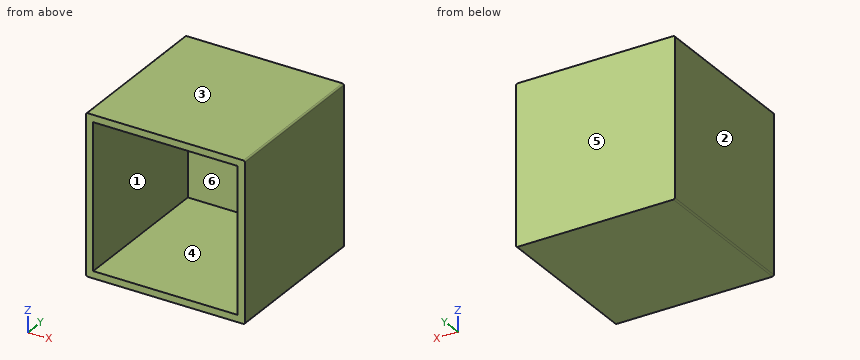
from build123d import *

# Parameters (mm, degrees)
F0_W     = 61.1250735819
F0_H     = 72.7862343192
F1_DEPTH = 28.448
F2_DEPTH = 32.6771
F3_DEPTH = 41.03624
F4_R     = 0.254
F5_T     = -1.27
F6_DEPTH = 3.302


with BuildPart() as f1:
    # F0 (on Top) → F1 (new body)
    with BuildSketch(Plane.XY):
        Rectangle(F0_W, F0_H)
    extrude(amount=F1_DEPTH)

    # F2 (cut): a face of the model
    f2_faces = [f1.faces().sort_by_distance(p)[0] for p in [
        (30.562536791, 0, 14.224),
    ]]
    extrude(f2_faces, amount=-F2_DEPTH, mode=Mode.SUBTRACT)

    # F3 (cut): a face of the model
    f3_faces = [f1.faces().sort_by_distance(p)[0] for p in [
        (-16.33855, -36.3931171596, 14.224),
    ]]
    extrude(f3_faces, amount=-F3_DEPTH, mode=Mode.SUBTRACT)

    # F4
    f4_edges = [f1.edges().sort_by_distance(p)[0] for p in [
        (-2.114563, 20.51812, 28.448),
        (-30.562537, 20.51812, 28.448),
        (-2.114563, 20.51812, 0),
        (-30.562537, 20.51812, 0),
    ]]
    fillet(f4_edges, radius=F4_R)

    # F5
    f5_openings = [f1.faces().sort_by_distance(p)[0] for p in [
        (-16.33855, 4.643123, 14.224),
    ]]
    offset(amount=F5_T, openings=f5_openings)

    # F6 (cut): a face of the model
    f6_faces = [f1.faces().sort_by_distance(p)[0] for p in [
        (-16.33855, 4.6431228404, 0.4023152874),
    ]]
    extrude(f6_faces, amount=-F6_DEPTH, mode=Mode.SUBTRACT)


solid = f1.part
Design review of the part built by this model. Coordinates are the model's own, in mm. Face numbers are marked on the shaded views. A direction names the side the tool comes from. Coordinates: 2 decimals unless noted, no trailing zeros. Order: outer loops, then holes, each group sorted by start corner. A loop starts at its lowest first (then second) coordinate and runs counter-clockwise, first axis right, second up. Notation, with made-up numbers: (3, 2) -> (19, 2) arc R19 ccw to (19, 23) -> close; hole circle Ø5 at (10, 2). An arc over 180 degrees is marked (long way). One line per item, written item: value.
1) We need section B-B, the plane z = 18. Give the boundary of the cut face in (x, y).
Output values:
outline: (-30.56, 7.95) -> (-29.29, 7.95) -> (-29.29, 35.12) -> (-3.38, 35.12) -> (-3.38, 7.95) -> (-2.11, 7.95) -> (-2.11, 36.39) -> (-30.56, 36.39) -> close
2) Machinability: for the marked faces 5 and 6, which of the approach directions +Z, -Z, +X, -X, +Y, -Y give a long, thin tool a straight path to every point of the face, cutting with its end or side? Answer none if there is none.
Output values:
face 5: +Z, -Z, +X, -X, +Y
face 6: -Y
3) Draft analysis for pull direction X (two halves, no side actions). For the marked faces 1, 2, 3 and 4, state which applies: +X half, -X half, draft (parallel to the pull), parting line (faces both ways), or undercut.
Output values:
face 1: undercut
face 2: -X half
face 3: draft
face 4: undercut
4) To check wall thickness, follow probe 1 along Z at (x, y) = (-26.5, 20.5); probe 2 along X at (y, z) = (17.25, 18.75); probe 3 along Y at (x, z) = (-14, 10). State the ranges of each line that lie inside material, in increasing order. Write a range as [from, to].
Output values:
probe 1: z = [0, 1.27], [27.18, 28.45]
probe 2: x = [-30.56, -29.29], [-3.38, -2.11]
probe 3: y = [35.12, 36.39]
5) Clearance check with a flat-ended pin moving along its axis: P1, Ø3, axis at x = -15, z = 9.5, coming from the -Y side. State where the tip first meets the part, or that it passes through.
Output values:
P1: stops at y = 35.12
6) We need section C-C, the plane x = -9.75. Give the boundary of the cut face in (y, z).
Output values:
outline: (7.95, 0) -> (36.39, 0) -> (36.39, 28.45) -> (7.95, 28.45) -> (7.95, 27.18) -> (35.12, 27.18) -> (35.12, 1.27) -> (7.95, 1.27) -> close
7) We need section A-A, the plane y = 27. Give the boundary of the cut face in (x, z), then the cut area to 3 significant figures.
Output values:
outline: (-30.56, 0.25) arc R0.25 ccw to (-30.31, 0) -> (-2.37, 0) arc R0.25 ccw to (-2.11, 0.25) -> (-2.11, 28.19) arc R0.25 ccw to (-2.37, 28.45) -> (-30.31, 28.45) arc R0.25 ccw to (-30.56, 28.19) -> close; hole (-29.29, 1.27) -> (-3.38, 1.27) -> (-3.38, 27.18) -> (-29.29, 27.18) -> close
area: 138 mm2
